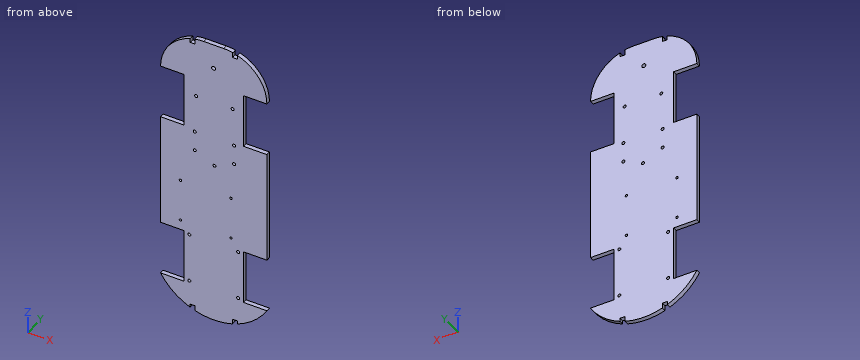
Autodesk Inventor part; units mm, degrees
ref_plane "YZ Plane" through (0, 0, 0) normal (1, 0, 0) x (0, 1, 0)
ref_plane "XZ Plane" through (0, 0, 0) normal (0, 1, 0) x (-1, 0, 0)
ref_plane "XY Plane" through (0, 0, 0) normal (0, 0, 1) x (1, 0, 0)
sketch "Sketch1" plane through (0, 0, 0) normal (0, 1, 0) x (-1, 0, 0)
  line L0 (-11.6621, 194.9999) -> (11.3379, 194.9999)
  line L1 (60.8379, 145.4999) -> (60.8379, -109.9001)
  line L2 (-61.1621, -109.9001) -> (-61.1621, 145.4999)
  line L3 (-61.1621, 194.9999) -> (61.1621, -194.9999) construction
  line L4 (60.8379, 194.9999) -> (-60.8379, -194.9999) construction
  arc A0 (60.8379, 145.4999) -> (11.3379, 194.9999) centre (11.3379, 145.4999) ccw
  arc A1 (-11.6621, 194.9999) -> (-61.1621, 145.4999) centre (-11.6621, 145.4999) ccw
  line L5 (-61.1621, 145.4999) -> (-34.3621, 145.4999)
  line L6 (-34.3621, 145.4999) -> (-34.3621, 82.9999)
  line L7 (-34.3621, 82.9999) -> (-61.1621, 82.9999)
  line L8 (-61.1621, 82.9999) -> (-61.1621, 145.4999)
  line L9 (-61.1621, 82.9999) -> (-61.1621, -47.4001)
  line L10 (-61.1621, -47.4001) -> (-34.3621, -47.4001)
  line L11 (-34.3621, -47.4001) -> (-34.3621, -109.9001)
  line L12 (-34.3621, -109.9001) -> (-61.1621, -109.9001)
  line L13 (-61.1621, -109.9001) -> (-61.1621, -47.4001)
  line L14 (60.8379, 145.4999) -> (34.0379, 145.4999)
  line L15 (34.0379, 145.4999) -> (34.0379, 82.9999)
  line L16 (34.0379, 82.9999) -> (60.8379, 82.9999)
  line L17 (60.8379, 82.9999) -> (60.8379, 145.4999)
  line L18 (60.8379, -47.4001) -> (34.0379, -47.4001)
  line L19 (34.0379, -47.4001) -> (34.0379, -109.9001)
  line L20 (34.0379, -109.9001) -> (60.8379, -109.9001)
  line L21 (60.8379, -109.9001) -> (60.8379, -47.4001)
  arc A2 (-61.1621, -109.9001) -> (60.8379, -109.9001) centre (-0.1621, -73.7641) ccw
  point P0 (0, 0)
  dimension "d0" = 122
  dimension "d1" = 390
  dimension "d2" = 49.5
  dimension "d4" = 26.8
  dimension "d5" = 62.5
  dimension "d6" = 130.4
  dimension "d7" = 26.8
  dimension "d8" = 62.5
  dimension "d9" = 26.8
  dimension "d10" = 62.5
  dimension "d11" = 26.8
  dimension "d12" = 62.5
  dimension "d13" = 70.9
extrude "Extrusion1" add sketch "Sketch1" along normal blind 5 contours L0 A0 L14 L15 L16 L1 L18 L19 L20 A2 L12 L11 L10 L2 L7 L6 L5 A1
sketch "Boceto2" plane through (0, 5, 0) normal (0, 1, 0) x (1, 0, 0)
  point P0 (0, 0)
sketch "Boceto3" plane through (0, 5, 0) normal (0, 1, 0) x (1, 0, 0)
  line L0 (-11.3379, -194.9999) -> (11.6621, -194.9999)
  line L1 (0.1621, -194.9999) -> (0.1621, -184.9999)
  line L2 (-2.7008, -183.6215) -> (19.0062, -183.6215)
  line L3 (19.0062, -183.6215) -> (-18.9938, -183.6215)
  line L4 (-2.7008, -148.6215) -> (19.0062, -148.6215)
  line L5 (19.0062, -148.6215) -> (-18.9938, -148.6215)
  line L6 (-18.9938, -148.6215) -> (-18.9938, -183.6215)
  line L7 (19.0062, -148.6215) -> (19.0062, -183.6215)
  line L8 (61.1621, -82.9999) -> (61.1621, 47.4001)
  line L9 (-60.8379, 47.4001) -> (-60.8379, -82.9999)
  line L10 (21.7666, -187.8715) -> (27.3666, -187.8715)
  line L11 (27.3666, -187.8715) -> (27.3666, -193.8715)
  line L12 (27.3666, -193.8715) -> (21.7666, -193.8715)
  line L13 (21.7666, -193.8715) -> (21.7666, -187.8715)
  line L14 (-11.3379, -194.9999) -> (-14.1379, -194.9999)
  arc A0 (-60.8379, -145.4999) -> (-11.3379, -194.9999) centre (-11.3379, -145.4999) ccw
  line L15 (-26.8363, -187.8801) -> (-21.2363, -187.8801)
  line L16 (-21.2363, -187.8801) -> (-21.2363, -193.8801)
  line L17 (-21.2363, -193.8801) -> (-26.8363, -193.8801)
  line L18 (-26.8363, -193.8801) -> (-26.8363, -187.8801)
  line L19 (21.7169, 135.4811) -> (27.3169, 135.4811)
  arc A1 (61.1621, 109.9001) -> (-60.8379, 109.9001) centre (0.1621, 73.7641) ccw
  line L20 (21.6786, 141.4811) -> (27.2786, 141.4811)
  line L21 (27.2786, 141.4811) -> (27.2786, 135.4811)
  line L22 (27.2786, 135.4811) -> (21.6786, 135.4811)
  line L23 (21.6786, 135.4811) -> (21.6786, 141.4811)
  line L24 (-26.9249, 141.4803) -> (-21.3249, 141.4803)
  line L25 (-21.3249, 141.4803) -> (-21.3249, 135.4803)
  line L26 (-21.3249, 135.4803) -> (-26.9249, 135.4803)
  line L27 (-26.9249, 135.4803) -> (-26.9249, 141.4803)
  line L28 (0.404, 144.7464) -> (0.404, -197.1126)
  line L29 (-34.0379, 47.4001) -> (-60.8379, 47.4001)
  line L30 (-60.8379, 47.4001) -> (-50.8379, 47.4001)
  line L31 (-41.5224, -16.7155) -> (-41.5224, 39.2845)
  line L32 (-41.5224, 39.2845) -> (43.4776, 39.2845)
  line L33 (43.4776, 39.2845) -> (43.4776, -16.7155)
  line L34 (43.4776, -16.7155) -> (-41.5224, -16.7155)
  line L35 (0.544, 11.7839) -> (0.544, 15.8925)
  line L36 (0.9776, 39.2845) -> (0.9776, -16.7155)
  line L37 (-21.3249, 141.4803) -> (21.6751, 141.4803)
  arc A2 (-60.8379, -145.4999) -> (-11.3379, -194.9999) centre (-11.3379, -145.4999) ccw
  line L38 (-34.0379, -82.9999) -> (-34.0379, -145.4999)
  line L39 (-21.2334, -193.8715) -> (-21.2169, -197.8147)
  line L40 (21.1268, -127.3043) -> (21.1268, -110.8043)
  line L41 (21.9297, -127.1387) -> (21.9297, -124.1387)
  line L42 (21.9297, -124.1387) -> (-19.9703, -124.1387)
  circle A3 centre (21.9297, -124.1387) radius 1.75
  circle A4 centre (-19.9703, -124.1387) radius 1.75
  line L43 (0.9797, -124.1387) -> (0.9776, -46.1387)
  circle A5 centre (0.9776, -46.1387) radius 1.75
  line L44 (3.2596, -48.0861) -> (0.432, -49.0887)
  line L45 (0.432, -49.0887) -> (-1.8499, -47.1412)
  line L46 (-1.8499, -47.1412) -> (-1.3044, -44.1913)
  line L47 (-1.3044, -44.1913) -> (1.5231, -43.1887)
  line L48 (1.5231, -43.1887) -> (3.8051, -45.1361)
  line L49 (3.8051, -45.1361) -> (3.2596, -48.0861)
  line L50 (0.9777, -49.2626) -> (28.4777, -49.2619)
  line L51 (28.4777, -49.2619) -> (-26.5223, -49.2619)
  line L52 (-26.5223, -49.2619) -> (-26.5223, -87.0619)
  line L53 (-26.5223, -87.0619) -> (28.4777, -87.0619)
  line L54 (28.4777, -87.0619) -> (28.4777, -49.2619)
  line L55 (-26.5223, -49.2619) -> (-23.3223, -49.2619)
  line L56 (-23.3223, -49.2619) -> (-23.3223, -54.9619)
  line L57 (-23.3223, -54.9619) -> (-21.5723, -54.9619)
  line L58 (-21.5723, -54.9619) -> (-21.5723, -56.7119)
  circle A6 centre (-21.5723, -56.7119) radius 1.75
  line L59 (-21.5723, -56.7119) -> (28.4777, -56.7119)
  line L60 (-21.5723, -56.7119) -> (-21.5723, -87.0619)
  line L61 (28.4777, -87.0619) -> (23.5277, -87.0619)
  line L62 (23.5277, -87.0619) -> (23.5277, -79.6119)
  circle A7 centre (23.5277, -79.6119) radius 1.75
  line L63 (23.5277, -79.6119) -> (-26.5223, -79.6119)
  line L64 (23.5277, -79.6119) -> (23.5277, -49.2619)
  circle A8 centre (23.5277, -56.7119) radius 1.75
  circle A9 centre (-21.5723, -79.6119) radius 1.75
  line L65 (-18.9938, -183.6215) -> (0.0062, -183.6215)
  line L66 (0.0062, -183.6215) -> (0.0062, -148.6215)
  line L67 (-21.2334, -193.8715) -> (21.7666, -193.8715)
  circle A10 centre (0.0062, -166.1215) radius 2.3
  line L68 (-41.5224, 39.2845) -> (-38.0224, 39.2845)
  line L69 (-38.0224, 39.2845) -> (-38.0224, 35.7845)
  line L70 (-38.0224, 35.7845) -> (19.9776, 35.7845)
  line L71 (19.9776, 35.7845) -> (19.9776, -13.2155)
  line L72 (19.9776, -13.2155) -> (-38.0224, -13.2155)
  line L73 (-38.0224, -13.2155) -> (-38.0224, 35.7845)
  circle A11 centre (-38.0224, 35.7845) radius 1.4
  circle A12 centre (19.9776, 35.7845) radius 1.4
  circle A13 centre (19.9776, -13.2155) radius 1.4
  circle A14 centre (-38.0224, -13.2155) radius 1.4
  line L74 (-34.0379, 109.9001) -> (-31.8379, 109.9001)
  line L75 (34.3621, 47.4001) -> (34.3621, 109.9001)
  line L76 (34.3621, 109.9001) -> (32.1621, 109.9001)
  line L77 (-31.8379, 109.9001) -> (32.1621, 109.9001)
  line L78 (32.1621, 109.9001) -> (32.1621, 47.4001)
  line L79 (32.1621, 47.4001) -> (-31.8379, 47.4001)
  line L80 (-31.8379, 47.4001) -> (-31.8379, 109.9001)
  line L81 (-31.8379, 109.9001) -> (-27.8379, 109.9001)
  line L82 (-27.8379, 109.9001) -> (-27.8379, 106.9001)
  line L83 (-27.8379, 106.9001) -> (28.1621, 106.9001)
  line L84 (28.1621, 106.9001) -> (28.1621, 49.9001)
  line L85 (28.1621, 49.9001) -> (-27.8379, 49.9001)
  line L86 (-27.8379, 49.9001) -> (-27.8379, 106.9001)
  circle A15 centre (-27.8379, 106.9001) radius 1.75
  circle A16 centre (28.1621, 106.9001) radius 1.75
  circle A17 centre (-27.8379, 49.9001) radius 1.75
  circle A18 centre (28.1621, 49.9001) radius 1.75
  point P0 (-21.5954, -147.627)
  point P1 (-17.4759, -197.9035)
  point P2 (-17.3346, -191.9653)
  point P3 (21.8949, -190.8298)
  point P4 (-20.3189, 140.8602)
  point P5 (0.404, -148.6215)
  point P6 (21.7169, 135.4811)
  point P7 (27.2786, 135.4811)
  point P8 (-26.8363, -192.5111)
  point P9 (-21.2363, -194.0001)
  point P10 (0.404, -148.6215)
  point P11 (-21.8071, -193.8801)
  point P12 (0.404, -183.6215)
  dimension "d16" = 10
  dimension "d18" = 38
  dimension "d19" = 35
  dimension "d21" = 38
  dimension "d29" = 5.6
  dimension "d30" = 6
  dimension "d36" = 5.6
  dimension "d44" = 5.6
  dimension "d45" = 6
  dimension "d46" = 5.6
  dimension "d47" = 6
  dimension "d69" = 56
  dimension "d70" = 85
  dimension "d128" = 16.5
  dimension "d133" = 3
  dimension "d134" = 3.5
  dimension "d135" = 3.5
  dimension "d136" = 78
  dimension "d137" = 41.9
  dimension "d138" = 3.5
  dimension "d139" = 3
  dimension "d140" = 27.5
  dimension "d141" = 55
  dimension "d142" = 37.8
  dimension "d143" = 3.2
  dimension "d144" = 5.7
  dimension "d146" = 1.75
  dimension "d147" = 1.75
  dimension "d148" = 3.5
  dimension "d149" = 4.95
  dimension "d150" = 7.45
  dimension "d151" = 3.5
  dimension "d152" = 3.5
  dimension "d153" = 3.5
  dimension "d156" = 19
  dimension "d157" = 35
  dimension "d158" = 90
  dimension "d159" = 43
  dimension "d160" = 43
  dimension "d161" = 4.6
  dimension "d164" = 3.5
  dimension "d165" = 3.5
  dimension "d166" = 58
  dimension "d167" = 49
  dimension "d168" = 58
  dimension "d169" = 90
  dimension "d170" = 2.8
  dimension "d171" = 2.8
  dimension "d172" = 2.8
  dimension "d173" = 2.8
  dimension "d174" = 2.2
  dimension "d175" = 2.2
  dimension "d176" = 62.5
  dimension "d177" = 64
  dimension "d178" = 4
  dimension "d179" = 3
  dimension "d180" = 56
  dimension "d181" = 57
  dimension "d182" = 3.5
  dimension "d183" = 3.5
  dimension "d184" = 3.5
  dimension "d185" = 3.5
extrude "Extrusión2" add sketch "Boceto3" against normal blind 1 contours L2 L66 A10 L28 | L28 A10 L4 L7 L2 | L2 L3 L6 L5 L4 L66 A10 | A10 L66 L28 | L28 A10 | A10 L66 | A10 L66 L4 L28
extrude "Extrusión4" cut sketch "Boceto3" against normal blind 20 contours L17 L18 A0 | A0 L18 L15 L16 L17 | L23 L20 L21 A1 | A1 L21 L19 L22 L23 | L13 L10 L11 L12 | L25 L26 L27 A1 | A1 L27 L24 L25
extrude "Extrusión6" cut sketch "Boceto3" against normal blind 10 contours A14 L73 L72 | L72 L73 A14 | A11 L73 L70 | L70 L69 A11 | A13 L71 L72 | L72 L71 A13 | L73 A11 L69 | A12 L71 L70 | L70 L71 A12
extrude "Extrusión7" cut sketch "Boceto3" against normal blind 5 contours A4 | A3 L40 L42 | L42 L40 A3 | A9 L60 L63 | L63 L60 A9 | A9 L63 L60 | L42 L41 A3 L40 | L40 A3 L41 L42 | L59 L58 A6 | A6 L60 L59 | L63 L62 A7 | A7 L64 L63 | L63 A9 L60 | L62 L64 A7 | L58 L60 A6 | A8 L64 L59 | L59 L64 A8 | A5 L28 | L28 A5 | L64 A8 L59 | L59 A8 L64
extrude "Extrusión8" cut sketch "Boceto3" against normal blind 5 contours A10 L66 L28 | L28 A10 | A10 L66
extrude "Extrusión9" cut sketch "Boceto3" against normal blind 10 contours A18 L84 L85 | L85 L84 A18 | A17 L86 L85 | L85 L86 A17 | A15 L86 L83 | L83 L82 A15 | A16 L84 L83 | L83 L84 A16 | L86 A15 L82
properties part number "base automodel"
Geometry: final body of the model. Coordinates: model frame, mm. Coordinates: 2 decimals unless noted, no trailing zeros. Loops run counter-clockwise (first coordinate to the right, second up) from the corner with the lowest first, then second, coordinate; pieces in that order, holes last. Notation, with made-up numbers: M 4,73.5 L 50,73.5 A4 ccw 50,78.5 Z; hole C 79.5,79.5 d7. An arc over 180 degrees is marked long. One line per item, written item: value. Start each with the question number.
1) Material intervals for L1, parallel to X at y = 4.25, z = -36; L2, parallel to Z at x = -46.5, y = 0.25; L3, parallel to Z at x = -53, y = 2, sorted ascending. Write a range as from..to.
2) Cut plane A-A (x = 54). Return loops of the section in (y, z), then the cut area to 3 significant figures.
3) Cut plane B-B (z = 106.5). Return loops of the section in (x, y), then the cut area to 3 significant figures.
4) Pin query (flat end, axial travel): P1, Ø1.5, axis at y = 4.5, z = -106, coming from the -X side; P2, Ø2.5, axis at y = 1.5, z = -138, coming from the -X side; P3, Ø2, axis at x = 28.16, z = -106.9, coming from the +Y side; P4, Ø0.5, axis at x = -21.5, y = 2, coming from the -Z side. Return the tip coordinate at first contact, or that it passes through.
5) Cut plane C-C (y = 1.6). Count the separate pieces of the cut face and the enclosed holes in it, then the cut area to 3 significant figures.
Evaluation:
1. L1: -60.84..-39.41, -36.64..18.59, 21.36..61.16
1. L2: -127.14..-109.9, -47.4..83, 145.5..180.34
1. L3: -120.67..-109.9, -47.4..83, 145.5..172.23
2. outline: M 0,-119.9 L 5,-119.9 L 5,-109.9 L 0,-109.9 Z; M 0,-47.4 L 5,-47.4 L 5,83 L 0,83 Z; M 0,145.5 L 5,145.5 L 5,171.15 L 0,171.15 Z
2. area: 830 mm^2
3. outline: M -34.04,0 L 34.36,0 L 34.36,5 L -34.04,5 Z
3. area: 342 mm^2
4. P1: x = -34.04
4. P2: x = -32.39
4. P3: through
4. P4: z = -141.35
5. separate pieces: 1
5. enclosed holes: 16
5. area: 32,200 mm^2
